from build123d import *

# Parameters (mm, degrees)
BOSS_EXTRUDE1_DEPTH = 0.8
BOSS_EXTRUDE2_DEPTH = 5


with BuildPart() as part:
    # Sketch1 → Boss-Extrude1 (new body)
    with BuildSketch(Plane(origin=(0, 0, 0), x_dir=(1, 0, 0), z_dir=(0, 1, 0))):
        with BuildLine():
            Line((31.85, 47), (-31.85, 47))
            ThreePointArc((-31.85, 47), (-34.85520382, 45.75520382), (-36.1, 42.75))
            Line((-36.1, 42.75), (-36.1, -42.75))
            ThreePointArc((-36.1, -42.75), (-34.85520382, -45.75520382), (-31.85, -47))
            Line((-31.85, -47), (31.85, -47))
            ThreePointArc((31.85, -47), (34.85520382, -45.75520382), (36.1, -42.75))
            Line((36.1, -42.75), (36.1, 42.75))
            ThreePointArc((36.1, 42.75), (34.85520382, 45.75520382), (31.85, 47))
        make_face()
        with BuildLine():
            Line((35.35, -42.75), (35.35, 42.75))
            ThreePointArc((35.35, 42.75), (34.324873734, 45.224873734), (31.85, 46.25))
            Line((31.85, 46.25), (-31.85, 46.25))
            ThreePointArc((-31.85, 46.25), (-34.324873734, 45.224873734), (-35.35, 42.75))
            Line((-35.35, 42.75), (-35.35, -42.75))
            ThreePointArc((-35.35, -42.75), (-34.324873734, -45.224873734), (-31.85, -46.25))
            Line((-31.85, -46.25), (31.85, -46.25))
            ThreePointArc((31.85, -46.25), (34.324873734, -45.224873734), (35.35, -42.75))
        make_face(mode=Mode.SUBTRACT)
    extrude(amount=-BOSS_EXTRUDE1_DEPTH)

    # Sketch2 → Boss-Extrude2 (add)
    with BuildSketch(Plane.XZ.offset(0.8)):
        with BuildLine():
            Line((36.1, -42.75), (36.1, 42.75))
            ThreePointArc((36.1, 42.75), (34.85520382, 45.75520382), (31.85, 47))
            Line((31.85, 47), (-31.85, 47))
            ThreePointArc((-31.85, 47), (-34.85520382, 45.75520382), (-36.1, 42.75))
            Line((-36.1, 42.75), (-36.1, -42.75))
            ThreePointArc((-36.1, -42.75), (-34.85520382, -45.75520382), (-31.85, -47))
            Line((-31.85, -47), (31.85, -47))
            ThreePointArc((31.85, -47), (34.85520382, -45.75520382), (36.1, -42.75))
        make_face()
        with BuildLine():
            Line((-34.6, 42.75), (-34.6, -42.75))
            ThreePointArc((-34.6, -42.75), (-33.794543648, -44.694543648), (-31.85, -45.5))
            Line((-31.85, -45.5), (31.85, -45.5))
            ThreePointArc((31.85, -45.5), (33.794543648, -44.694543648), (34.6, -42.75))
            Line((34.6, -42.75), (34.6, 42.75))
            ThreePointArc((34.6, 42.75), (33.794543648, 44.694543648), (31.85, 45.5))
            Line((31.85, 45.5), (-31.85, 45.5))
            ThreePointArc((-31.85, 45.5), (-33.794543648, 44.694543648), (-34.6, 42.75))
        make_face(mode=Mode.SUBTRACT)
    extrude(amount=BOSS_EXTRUDE2_DEPTH)


solid = part.part
The listing builds one solid part. Answer for the finished solid, in the listing's coordinates (mm). A direction names the side the tool comes from. Coordinates: 2 decimals unless noted, no trailing zeros. Write each loop counter-clockwise with the first axis right and the second up, starting at its lowest first coordinate (ties: lowest second). Pieces come first, ordered by that corner, then holes. Notation, with made-up numbers: (28.5, 55.5) - (33.5, 55.5) arc R32 ccw to (33.5, 94.5) - close; hole circle Ø7 at (-26.5, 41.5). An arc over 180 degrees is marked (long way). Put each result on its own line as item: value.
1. The part is cut by section A-A on z = 3.5. Give the vertices of the cut face in (x, y), plus the area to 3 significant figures.
Answer sheet:
outline: (-36.1, -5.8) - (-34.6, -5.8) - (-34.6, -0.8) - (-35.35, -0.8) - (-35.35, 0) - (-36.1, 0) - close; (34.6, -5.8) - (36.1, -5.8) - (36.1, 0) - (35.35, 0) - (35.35, -0.8) - (34.6, -0.8) - close
area: 16.2 mm^2
2. The part is cut by section C-C on y = -3. Give the vertices of the cut face in (x, z), plus the area to 3 significant figures.
Answer sheet:
outline: (-36.1, -42.75) arc R4.25 ccw to (-31.85, -47) - (31.85, -47) arc R4.25 ccw to (36.1, -42.75) - (36.1, 42.75) arc R4.25 ccw to (31.85, 47) - (-31.85, 47) arc R4.25 ccw to (-36.1, 42.75) - close; hole (-34.6, -42.75) arc R2.75 ccw to (-31.85, -45.5) - (31.85, -45.5) arc R2.75 ccw to (34.6, -42.75) - (34.6, 42.75) arc R2.75 ccw to (31.85, 45.5) - (-31.85, 45.5) arc R2.75 ccw to (-34.6, 42.75) - close
area: 481 mm^2
3. Determine the mould class of faces 1 (the face through (-34.6, -3, 1)), 2 (the face through (34.82, -2.86, -45.79)), 3 (the face through (-35, -5.8, 0)) for opening direction X: pulls with the +X half, pulls with the -X half, needs draft (parallel to the pull), parting line crosses it, or undercut.
Answer sheet:
face 1: undercut
face 2: pulls with the +X half
face 3: needs draft
4. Find the intervals of material crossed by line 1 along X through (y, z) = (-5.5, -39); line 2 along Z through (x, y) = (-3.5, -4.9); line 3 along Z through (x, y) = (-28, -0.6), in increasing order. Write a range as from..to.
Answer sheet:
line 1: x = -36.1..-34.6, 34.6..36.1
line 2: z = -47..-45.5, 45.5..47
line 3: z = -47..-46.25, 46.25..47
5. The part is cut by section B-B on x = -12.5. Give the vertices of the cut face in (y, z), plus the area to 3 significant figures.
Answer sheet:
outline: (-5.8, -47) - (0, -47) - (0, -46.25) - (-0.8, -46.25) - (-0.8, -45.5) - (-5.8, -45.5) - close; (-5.8, 45.5) - (-0.8, 45.5) - (-0.8, 46.25) - (0, 46.25) - (0, 47) - (-5.8, 47) - close
area: 16.2 mm^2
6. A tool of negligible diameter and unlimited length cuts with its end or side. For faces 4 (the face through (34.35, -0.39, -45.2)), 5 (the face through (0, -3, 47)), 6 (the face through (0, -3, 45.5)), from which of +Z, -Z, +X, -X, +Y, -Y can it reach the whole face along a straight path? Write none if from no direction.
Answer sheet:
face 4: +Y
face 5: +Z, +X, -X, +Y, -Y
face 6: +Y, -Y
